Input: part model. Units: mm. Frame: model coordinates. A direction names the side the tool comes from. Coordinates: 2 decimals unless noted, no trailing zeros. Order: outer loops, then holes, each group sorted by start corner. A loop starts at its lowest first (then second) coordinate and runs counter-clockwise, first axis right, second up. Notation, with made-up numbers: M 78,-8.5 L 96,-8.5 A12 cw 96,10.5 Z; hole C 13,0.5 d3. An arc over 180 degrees is marked long. Answer in a Markdown table with one row per item.
from build123d import *

# Parameters (mm, degrees)
BOSS_EXTRUDE1_DEPTH = 3.175
SKETCH2_R           = 1.524
CUT_EXTRUDE1_DEPTH  = 3.175


with BuildPart() as part:
    # Sketch1 → Boss-Extrude1 (new body)
    with BuildSketch(Plane.XY):
        with BuildLine():
            Line((-2.54, 0), (-6.985, 0))
            ThreePointArc((-6.985, 0), (-8.781051224, 0.743948776), (-9.525, 2.54))
            Line((-9.525, 2.54), (-9.525, 38.1))
            ThreePointArc((-9.525, 38.1), (-4.7625, 52.231044912), (0, 38.1))
            Line((0, 38.1), (0, 2.54))
            ThreePointArc((0, 2.54), (-0.743948776, 0.743948776), (-2.54, 0))
        make_face()
    extrude(amount=BOSS_EXTRUDE1_DEPTH)

    # Sketch2 → Cut-Extrude1 (cut)
    with BuildSketch(Plane.XY.offset(3.175)):
        with Locations((-4.7625, 44.362984272)):
            Circle(SKETCH2_R)
    extrude(amount=-CUT_EXTRUDE1_DEPTH, mode=Mode.SUBTRACT)


solid = part.part
1) Contact query for flat-ended pins moving along their axis: pin 1 (1 mm diameter, centred on x = -1, z = 1.5, fed in from +Y); pin 2 (1.6 mm diameter, centred on y = 25.5, z = 2, fed in from -X) (3 decimals). Output: stop coordinate, or through.
Resolved:
| item | result |
|---|---|
| pin 1 | stops at y = 51.52 |
| pin 2 | stops at x = -9.525 |
2) Cut plane A-A, the plane z = 2.15. Output: boundary loops of the cut face in (x, y) (1 decimal), and give its area (3 significant figures).
Resolved:
| item | result |
|---|---|
| outline | M -9.5,2.5 A2.5 ccw -7,0 L -2.5,0 A2.5 ccw 0,2.5 L 0,38.1 A7.9 ccw long -9.5,38.1 Z; hole C -4.8,44.4 d3 |
| area | 537 mm2 |
3) Cut plane C-C, the plane y = 28.5. Output: boundary loops of the cut face in (x, z) (3 decimals), and give its area (3 significant figures).
Resolved:
| item | result |
|---|---|
| outline | M -9.525,0 L 0,0 L 0,3.175 L -9.525,3.175 Z |
| area | 30.2 mm2 |
4) Cut plane B-B, the plane x = -5.5. Output: boundary loops of the cut face in (y, z) (3 decimals), and give its area (3 significant figures).
Resolved:
| item | result |
|---|---|
| outline | M 0,0 L 43.029,0 L 43.029,3.175 L 0,3.175 Z; M 45.697,0 L 52.196,0 L 52.196,3.175 L 45.697,3.175 Z |
| area | 157 mm2 |
5) Material intervals for probe 1 along X at (y, z) = (19, 2.9) (3 decimals); probe 2 along Y at (x, z) = (-6, 0.6); probe 3 along Y at (x, z) = (-5.5, 1.7), sorted ascending.
Resolved:
| item | result |
|---|---|
| probe 1 | x = -9.525 to 0 |
| probe 2 | y = 0 to 43.47, 45.25 to 52.13 |
| probe 3 | y = 0 to 43.03, 45.7 to 52.2 |
6) Mould query, pull axis Y, two halves, no side actions, for faces 4 (the face through (-0.724, 0.764, 1.565)), 5 (the face through (-5.037, 52.226, 1.565)), 6 (the face through (-5.093, 42.875, 1.61)). Classes: +Y half, -Y half, draft (parallel to the pull), parting line (faces both ways), or undercut.
Resolved:
| item | result |
|---|---|
| face 4 | -Y half |
| face 5 | parting line |
| face 6 | undercut |
7) Cut plane D-D, the plane x = -11. Output: boundary loops of the cut face in (y, z) (3 decimals), and give its area (3 significant figures).
Resolved:
| item | result |
|---|---|
| outline | M 39.567,0 L 49.159,0 L 49.159,3.175 L 39.567,3.175 Z |
| area | 30.5 mm2 |
8) Reachability of faces 1 (the face through (-5, 26, 3.175)), 2 (the face through (-9.525, 20, 2)), 3 (the face through (0, 21, 2)) from +Z, -Z, +X, -X, +Y, -Y: full face, straight path, thin tool, end or side. Return the list, or none.
Resolved:
| item | result |
|---|---|
| face 1 | +Z, +X, -X, +Y, -Y |
| face 2 | +Z, -Z, -X, -Y |
| face 3 | +Z, -Z, +X, -Y |
